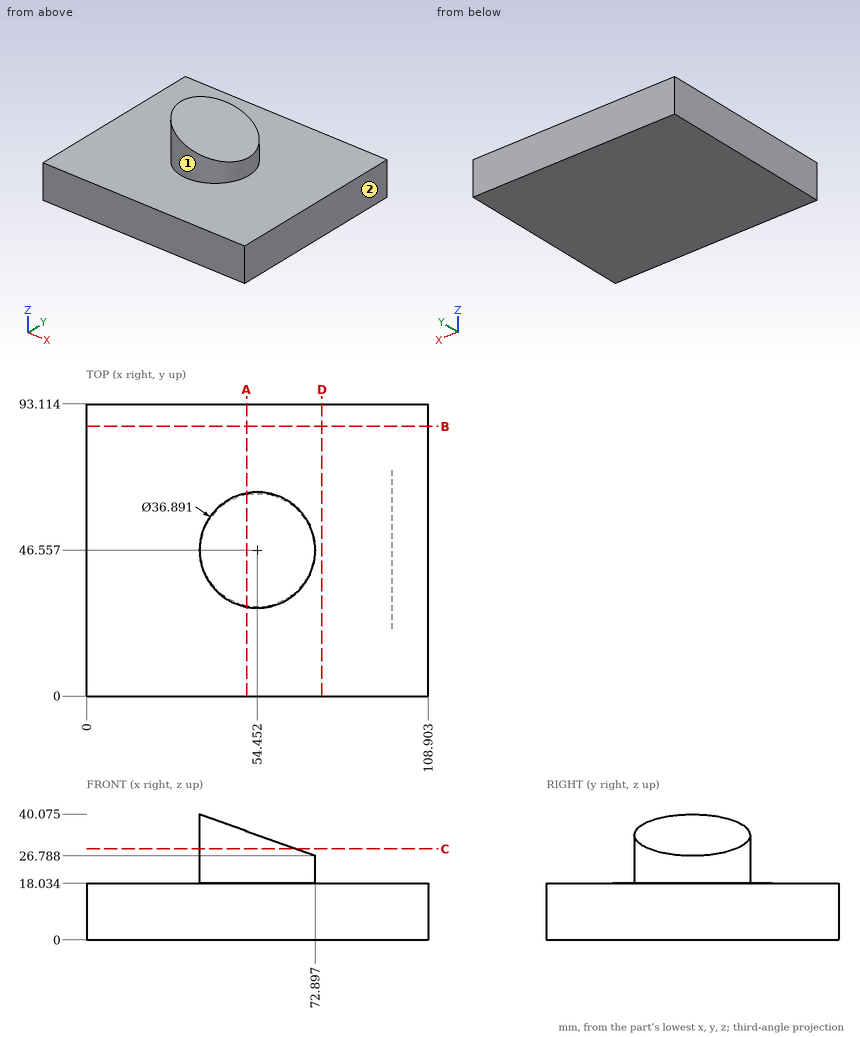
Verification items for this drawing (mm, ordinates from the low corner). A direction names the side the tool comes from. Coordinates: 2 decimals unless noted, no trailing zeros. Order: outer loops, then holes, each group sorted by start corner. A loop starts at its lowest first (then second) coordinate and runs counter-clockwise, first axis right, second up. Notation, with made-up numbers: (43.5, 53.5) -> (65.5, 53.5) arc R16 ccw to (65.5, 76.5) -> close; hole circle Ø3 at (17.5, -27.5). An arc over 180 degrees is marked (long way). Put each result on its own line as item: value. Start each with the question number.
1. Access from +Z, -Z, +X, -X, +Y, -Y to the whole of each face (thin tool, end or side, straight path). Record for the marked faces 1 and 2.
2. Cross-section at B-B, the plane y = 86. Record the boundary of the cut face in (x, z).
3. Cross-section at C-C, the plane z = 29. Record the boundary of the cut face in (x, y) (1 decimal).
4. Cross-section at D-D, the plane x = 75. Record the boundary of the cut face in (y, z).
5. Cross-section at A-A, the plane x = 51. Record the boundary of the cut face in (y, z) (1 decimal).
6. Go/stop test with flat-tipped pins: pin 1 Ø12 at (x, y) = (62, 68) entering from +Z; pin 2 Ø10 at (x, y) = (71, 36.5) entering from +Z; pin 3 Ø5 at (x, y) = (70.5, 14) entering from +Z. Record where each tip stops, or that it passes through.
7. Material ranges on L1, parallel to Z at x = 17, y = 38.5; L2, parallel to Y at x = 43, z = 29 (1 decimal); L3, parallel to Y at x = 52.5, z = 28 (1 decimal), recorded low to high. Write a range as [from, to].
Computed:
1. face 1: +Z
1. face 2: +Z, -Z, +X, +Y, -Y
2. outline: (0, 0) -> (108.9, 0) -> (108.9, 18.03) -> (0, 18.03) -> close
3. outline: (66.8, 32.8) -> (66.8, 60.3) arc R18.4 ccw (long way) to start
4. outline: (0, 0) -> (93.11, 0) -> (93.11, 18.03) -> (0, 18.03) -> close
5. outline: (0, 0) -> (93.1, 0) -> (93.1, 18) -> (64.7, 18) -> (64.7, 34.7) -> (28.4, 34.7) -> (28.4, 18) -> (0, 18) -> close
6. pin 1: z = 32.55
6. pin 2: z = 29.27
6. pin 3: z = 18.03
7. L1: [0, 18.03]
7. L2: [32.1, 61]
7. L3: [28.2, 64.9]
